Read the model definition and answer for the solid it produces. Units are mm, in the model's axes. A direction names the side the tool comes from. Coordinates: 2 decimals unless noted, no trailing zeros. Order: outer loops, then holes, each group sorted by start corner. A loop starts at its lowest first (then second) coordinate and runs counter-clockwise, first axis right, second up. Notation, with made-up numbers: (-34.5, 86) - (-24.5, 86) arc R11 ccw to (-24.5, 94) - close; hole circle Ø4 at (70, -23). An arc over 180 degrees is marked (long way). Write item = value, one per line.
from build123d import *

# Parameters (mm, degrees)
BOSS_EXTRUDE1_DEPTH = 10


with BuildPart() as part:
    # Sketch1 → Boss-Extrude1 (new body)
    with BuildSketch(Plane(origin=(0, 0, 0), x_dir=(1, 0, 0), z_dir=(0, 1, 0))):
        Polygon((0, -7.808777861), (6.7626, -3.90438893), (6.7626, 3.90438893), (0, 7.808777861), (-6.7626, 3.90438893), (-6.7626, -3.90438893), align=None)
        Polygon((5.5626, -3.211568607), (5.5626, 3.211568607), (0, 6.423137215), (-5.5626, 3.211568607), (-5.5626, -3.211568607), (0, -6.423137215), align=None, mode=Mode.SUBTRACT)
        with BuildLine():
            ThreePointArc((9.224161182, -6.935060385), (7.396240301, -3.679481838), (6.7626, -2.8e-08))
            Line((6.7626, -2.8e-08), (6.7626, -3.90438893))
            Line((6.7626, -3.90438893), (3.3813, -5.856583396))
            ThreePointArc((3.3813, -5.856583396), (6.501441474, -5.319266604), (9.224161182, -6.935060385))
        make_face()
        with BuildLine():
            ThreePointArc((6.7626, -2.8e-08), (7.396240292, 3.679481812), (9.224161182, 6.935060385))
            ThreePointArc((9.224161182, 6.935060385), (6.501441474, 5.319266604), (3.3813, 5.856583396))
            Line((3.3813, 5.856583396), (6.7626, 3.90438893))
            Line((6.7626, 3.90438893), (6.7626, -2.8e-08))
        make_face()
        with BuildLine():
            Line((24.126561031, 6.363961031), (25.540774593, 7.778174593))
            ThreePointArc((25.540774593, 7.778174593), (6.7626, 0), (25.540774593, -7.778174593))
            Line((25.540774593, -7.778174593), (24.126561031, -6.363961031))
            ThreePointArc((24.126561031, -6.363961031), (8.7626, 0), (24.126561031, 6.363961031))
        make_face()
    extrude(amount=BOSS_EXTRUDE1_DEPTH)


solid = part.part
1) Flat-ended cylindrical pins translate along their axes: pin 1 Ø1 at (x, y) = (13, 8) entering from +Z; pin 2 Ø5 at (y, z) = (5, 1.5) entering from +X; pin 3 Ø2 at (y, z) = (2.5, -8) entering from -X. Find the tip coordinate at first contact, or state that the pin passes through.
Returned:
pin_1 = 10.14
pin_2 = 9.7
pin_3 = -1.4
2) Determine the mould class of faces 1 (the face through (6.46, 4.93, 5.31)), 2 (the face through (-6.763, 5, 0)), 3 (the face through (24.84, 4.93, 7.08)) for opening direction X: pulls with the +X half, pulls with the -X half, needs draft (parallel to the pull), parting line crosses it, or undercut.
Returned:
face_1 = undercut
face_2 = pulls with the -X half
face_3 = pulls with the +X half
3) For faces 4 (the face through (1.667, 4.93, 6.846)), 5 (the face through (2.74, 4.93, 4.84)), 6 (the face through (1.71, 4.93, -6.82)), 7 (the face through (24.82, 4.93, -7.06)), determine the directions among +Z, -Z, +X, -X, +Y, -Y from which every point of the face is accessible in a straight line to the end or side of a thin tool.
Returned:
face_4 = +Z, +Y, -Y
face_5 = +Y, -Y
face_6 = -Z, +Y, -Y
face_7 = +X, +Y, -Y
4) The part is cut by section A-A (z = 0). Determine the outline of the cut face in (x, y).
Returned:
outline = (-6.76, 0) - (-5.56, 0) - (-5.56, 10) - (-6.76, 10) - close; (5.56, 0) - (8.76, 0) - (8.76, 10) - (5.56, 10) - close
5) The part is cut by section B-B (y = 8.25). Determine the outline of the cut face in (x, z).
Returned:
outline = (-6.76, -3.9) - (0, -7.81) - (3.38, -5.86) arc R4.58 cw to (9.22, -6.94) arc R11 ccw to (25.54, -7.78) - (24.13, -6.36) arc R9 cw (long way) to (24.13, 6.36) - (25.54, 7.78) arc R11 ccw to (9.22, 6.94) arc R4.58 cw to (3.38, 5.86) - (0, 7.81) - (-6.76, 3.9) - close; hole (-5.56, -3.21) - (0, -6.42) - (5.56, -3.21) - (5.56, 3.21) - (0, 6.42) - (-5.56, 3.21) - close
6) The part is cut by section C-C (x = 1.5). Determine the outline of the cut face in (y, z), and give its area (3 significant figures).
Returned:
outline = (0, -6.94) - (10, -6.94) - (10, -5.56) - (0, -5.56) - close; (0, 5.56) - (10, 5.56) - (10, 6.94) - (0, 6.94) - close
area = 27.7 mm^2
7) Straight lines are drawn through the part: line 1 along X through (y, z) = (9, -6.5); line 2 along X through (y, z) = (8, 7.25); line 3 along X through (y, z) = (8.25, -1.5). For each, find the intervals that lie inside material, in ascending order. Write a range as from..to.
Returned:
line_1 = -2.27..2.27, 8.82..11.54, 23.99..24.26
line_2 = -0.97..0.97, 9.49..12.43, 23.1..25.01
line_3 = -6.76..-5.56, 5.56..8.89
